Can you work these out from the drawing? Everything is in mm from the part's minimum corner. Coordinates: 2 decimals unless noted, no trailing zeros. Order: outer loops, then holes, each group sorted by start corner. A loop starts at its lowest first (then second) coordinate and runs counter-clockwise, first axis right, second up. Notation, with made-up numbers: M -12,74 L 29,74 A36 cw 29,111 Z; hole C -9.5,60 d9. An arc over 180 degrees is marked long. Answer as a JSON object with one key per item and string values.
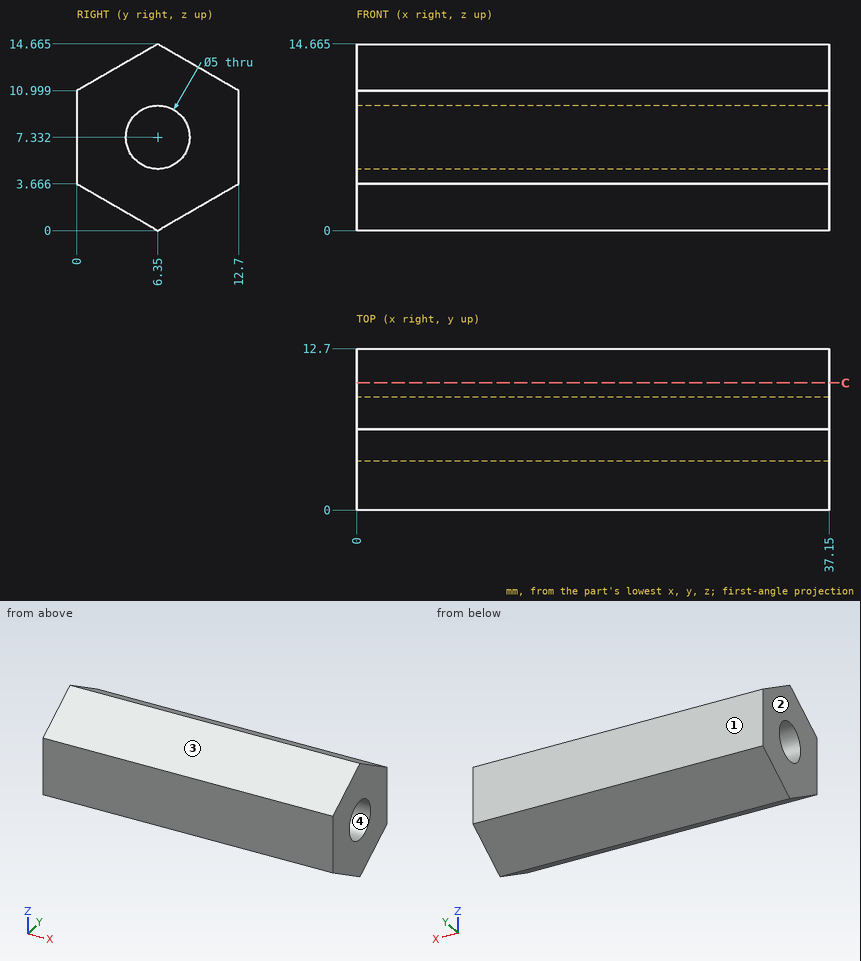
Item 1: I want a section at C-C, the plane y = 10. Write out the boundary of the cut face in (x, z).
Answers follow:
{"outline": "M 0,2.11 L 37.15,2.11 L 37.15,12.56 L 0,12.56 Z"}
Item 2: I'm going to push a flat-ended pin straight in: pin 1 (2 mm diameter, centred on x = 4, y = 2, fed in from +Z). Where does the tip first touch, or does it pass through?
Answers follow:
{"pin 1": "stops at z = 12.73"}
Item 3: If we mould it in two halves opening along Y, with no side actions, what happens to the marked faces 1, 2, 3 and 4? For each: pulls with the +Y half, pulls with the -Y half, needs draft (parallel to the pull), parting line crosses it, or undercut.
Answers follow:
{"face 1": "pulls with the +Y half", "face 2": "needs draft", "face 3": "pulls with the -Y half", "face 4": "undercut"}
Item 4: Please list where these lines run through material, in increasing order: line 1 (Y direction, x = 22, z = 9.25) (1 decimal); line 2 (Y direction, x = 33, z = 8.5); line 3 (Z direction, x = 35.5, y = 5) (1 decimal).
Answers follow:
{"line 1": "y = 0 to 4.7, 8 to 12.7", "line 2": "y = 0 to 4.14, 8.56 to 12.7", "line 3": "z = 0.8 to 5.2, 9.4 to 13.9"}
